For this review, take the finished solid that the model builds, in its own axes (mm). A direction names the side the tool comes from. Coordinates: 2 decimals unless noted, no trailing zeros. Write each loop counter-clockwise with the first axis right and the second up, starting at its lowest first coordinate (ties: lowest second). Pieces come first, ordered by that corner, then holes. Notation, with made-up numbers: (55.5, 2) -> (59.5, 2) arc R15 ccw to (59.5, 24) -> close; hole circle Ø9 at (-36, -12). An arc over 180 degrees is marked (long way). Put each result on its own line as item: value. Start each with the question number.
Item 1: For faces 5 (the flat face through (0, 4, 3.175)), 6 (the flat face through (30.185, 0.244, 24.031)), list the 3-axis set-ups (+Z, -Z, +X, -X, +Y, -Y) from which the entire face can be reached by the end or side of a thin tool; tool diameter is ignored.
Item 2: Consider section A-A on x = 0. Give the boundary of the cut face in (y, z) (1 decimal).
Item 3: Consider section D-D on y = 11.5. Give the boundary of the cut face in (x, z) (3 decimals).
Item 4: The part is to be moulded in two halves that separate along Y. For faces 1 (the cylindrical face through (2.43, 2.23, 1.57)), 2 (the flat face through (0, 17.462, 2)), 3 (the flat face through (28.575, -8, 16)), 4 (the flat face through (0, -17.462, 3)), say which applies: +Y half, -Y half, draft (parallel to the pull), parting line (faces both ways), or undercut.
Item 5: Insertion check: P1, Ø1, axis at y = -6.5, z = 32, coming from the -X side; P2, Ø2, axis at x = 0.5, y = -14, coming from the +Z side (3 decimals). Each pin has a flat end and moves straight along its axis. Give the tip position at first contact, or say it passes through.
Item 6: Consider section C-C on y = 1.5. Give the boundary of the cut face in (x, z) (3 decimals), and give its area (3 significant figures).
Item 7: To check wall thickness, follow L1, parallel to Y at x = 0, z = 1; L2, parallel to X at y = -16, z = 30.5 (3 decimals); L3, parallel to Z at x = 19.5, y = -9.5 (3 decimals). State the ranges of each line that lie inside material, in increasing order.
```python
from build123d import *

# Parameters (mm, degrees)
SKETCH2_W                    = 57.15
SKETCH2_H                    = 34.925
BASE_FLANGE1_DEPTH           = 3.175
EDGE_FLANGE1_STRIP_W         = 14.7
EDGE_FLANGE1_STRIP_H         = 3.175
EDGE_FLANGE1_STRIP_CUT_DEPTH = 34.925
EDGE_FLANGE1_DEPTH           = 34.925
CUT_EXTRUDE1_DEPTH           = 3.175
M6_CLEARANCE_HOLE1_D         = 6.6


# Sheet-metal steps are written as plain solids
with BuildPart() as part:
    # Sketch2 → Base-Flange1 (new body)
    with BuildSketch(Plane.XY):
        Rectangle(SKETCH2_W, SKETCH2_H)
    extrude(amount=BASE_FLANGE1_DEPTH)

    # Edge-Flange1 strip (across the edge) → Edge-Flange1 strip cut (cut)
    with BuildSketch(Plane(origin=(28.575, -17.4625, 3.175), x_dir=(-1, 0, 0), z_dir=(0, 1, 0))):
        with Locations((-6.35, -1.5875)):
            Rectangle(EDGE_FLANGE1_STRIP_W, EDGE_FLANGE1_STRIP_H)
    edge_flange1_strip_cut = extrude(amount=EDGE_FLANGE1_STRIP_CUT_DEPTH, mode=Mode.SUBTRACT)

    # Edge-Flange1 section (across the edge) → Edge-Flange1 (add)
    with BuildSketch(Plane(origin=(28.575, -17.4625, 3.175), x_dir=(-1, 0, 0), z_dir=(0, 1, 0))):
        with BuildLine():
            Line((-3.175, 1), (-3.175, 41.275))
            Line((-3.175, 41.275), (0, 41.275))
            Line((0, 41.275), (0, 1))
            ThreePointArc((0, 1), (0.292893219, 0.292893219), (1, 0))
            Line((1, 0), (1, -3.175))
            ThreePointArc((1, -3.175), (-1.952170811, -1.952170811), (-3.175, 1))
        make_face()
    edge_flange1 = extrude(amount=EDGE_FLANGE1_DEPTH)

    # Sketch10 → Cut-Extrude1 (cut)
    with BuildSketch(Plane(origin=(31.75, 0, 0), x_dir=(0, 0, -1), z_dir=(1, 0, 0))):
        Polygon((-4.175, 17.4625), (-44.45, -17.4625), (-44.45, 17.4625), align=None)
    cut_extrude1 = extrude(amount=-CUT_EXTRUDE1_DEPTH, mode=Mode.SUBTRACT)

    # Mirror1: Edge-Flange1 strip cut, Edge-Flange1, Cut-Extrude1 across plane
    add(edge_flange1_strip_cut.mirror(Plane(origin=(0, 0, 0), x_dir=(0, 0, 1), z_dir=(1, 0, 0))), mode=Mode.SUBTRACT)
    add(edge_flange1.mirror(Plane(origin=(0, 0, 0), x_dir=(0, 0, 1), z_dir=(1, 0, 0))))
    add(cut_extrude1.mirror(Plane(origin=(0, 0, 0), x_dir=(0, 0, 1), z_dir=(1, 0, 0))), mode=Mode.SUBTRACT)

    # M6 Clearance Hole1 (through all)
    with Locations(Plane.XY.offset(3.175)):
        with Locations((0, 0)):
            Hole(M6_CLEARANCE_HOLE1_D / 2)


solid = part.part
```
Return value:
1. face 5: +Z, +Y, -Y
1. face 6: +Z, +X, -X, +Y
2. outline: (-17.5, 0) -> (-3.3, 0) -> (-3.3, 3.2) -> (-17.5, 3.2) -> close; (3.3, 0) -> (17.5, 0) -> (17.5, 3.2) -> (3.3, 3.2) -> close
3. outline: (-31.75, 4.175) arc R4.175 ccw to (-27.575, 0) -> (27.575, 0) arc R4.175 ccw to (31.75, 4.175) -> (31.75, 11.051) -> (28.575, 11.051) -> (28.575, 4.175) arc R1 cw to (27.575, 3.175) -> (-27.575, 3.175) arc R1 cw to (-28.575, 4.175) -> (-28.575, 11.051) -> (-31.75, 11.051) -> close
4. face 1: undercut
4. face 2: +Y half
4. face 3: draft
4. face 4: -Y half
5. P1: x = -31.75
5. P2: z = 3.175
6. outline: (-31.75, 4.175) arc R4.175 ccw to (-27.575, 0) -> (-2.939, 0) -> (-2.939, 3.175) -> (-27.575, 3.175) arc R1 cw to (-28.575, 4.175) -> (-28.575, 22.583) -> (-31.75, 22.583) -> close; (2.939, 0) -> (27.575, 0) arc R4.175 ccw to (31.75, 4.175) -> (31.75, 22.583) -> (28.575, 22.583) -> (28.575, 4.175) arc R1 cw to (27.575, 3.175) -> (2.939, 3.175) -> close
6. area: 299 mm^2
7. L1: -17.46 to -3.3, 3.3 to 17.46
7. L2: -31.75 to -28.575, 28.575 to 31.75
7. L3: 0 to 3.175
